Read the model definition and answer for the solid it produces. Units are mm, in the model's axes. A direction names the side the tool comes from. Coordinates: 2 decimals unless noted, no trailing zeros. Write each loop counter-clockwise with the first axis right and the second up, starting at its lowest first coordinate (ties: lowest second). Pieces come first, ordered by that corner, then holes. Notation, with made-up numbers: (-0.75, -18.75) -> (40.25, -18.75) arc R20 ccw to (40.25, -2.75) -> close; hole circle Ø2 at (26.5, -27). An arc over 180 degrees is marked (long way). Answer in a Markdown table with one row per item. Add a question column.
Item 1: Given pin 1 Ø7.5 at (x, z) = (141, 517.5) entering from +Y; pin 2 Ø2 at (x, z) = (90, 215.5) entering from +Y, each flat-ended and moving along its own axis, determine where each tip first touches the part or whether it passes through.
Item 2: Straight lines are drawn through the part: line 1 (Z direction, x = 42, y = 195); line 2 (Y direction, x = 225, z = 163.5); line 3 (Z direction, x = 191, y = 358.5). For each, find the intervals that lie inside material, in ascending order. Write a range as from..to.
Item 3: For a pull along Z with two mould halves and no side action, classify faces 4 (the face through (188, 0, 263)), 5 (the face through (188, 175, 0)), 6 (the face through (188, 168, 533.4)) as +Z half, -Z half, draft (parallel to the pull), parting line (faces both ways), or undercut.
Item 4: Which of the six approach directions +Z, -Z, +X, -X, +Y, -Y give full straight-line access (tool end or side, diameter ignored) to faces 1 (the face through (188, 381, 13)), 2 (the face through (188, 193, 25.4)), 3 (the face through (188, 355.6, 521))?
Item 5: Section B-B on x = 97.5 is taken. Write down the section's boundary in (y, z), then the cut area to 3 significant figures.
Item 6: Section C-C on z = 370 is taken. Write down the section's boundary in (x, y), then the cut area to 3 significant figures.
Item 7: Section A-A on y = 272 is taken. Write down the section's boundary in (x, z), then the cut area to 3 significant figures.
```python
from build123d import *

# Parameters (mm, degrees)
F0_W     = 381
F0_H     = 381
F1_DEPTH = 25.4
F2_W     = 25.4
F2_H     = 508
F3_DEPTH = 381
F4_W     = 381
F4_H     = 355.6
F4_H_2   = 25.4
F5_DEPTH = 25.4


with BuildPart() as f1:
    # F0 (on Top) → F1 (new body)
    with BuildSketch(Plane.XY):
        with Locations((190.5, 190.5)):
            Rectangle(F0_W, F0_H)
    extrude(amount=F1_DEPTH)

    # F2 (on Right) → F3 (join)
    with BuildSketch(Plane.YZ):
        with Locations((-12.7, 254)):
            Rectangle(F2_W, F2_H)
    extrude(amount=F3_DEPTH)

    # F4 (on face) → F5 (join)
    with BuildSketch(Plane.XY.offset(508)):
        with Locations((190.5, 177.8)):
            Rectangle(F4_W, F4_H)
        with Locations((190.5, -12.7)):
            Rectangle(F4_W, F4_H_2)
    extrude(amount=F5_DEPTH)


solid = f1.part
```
Results below:
| question | item | result |
|---|---|---|
| 1 | pin 1 | stops at y = 355.6 |
| 1 | pin 2 | stops at y = 0 |
| 2 | line 1 | z = 0..25.4, 508..533.4 |
| 2 | line 2 | y = -25.4..0 |
| 2 | line 3 | z = 0..25.4 |
| 3 | face 4 | undercut |
| 3 | face 5 | -Z half |
| 3 | face 6 | +Z half |
| 4 | face 1 | +Z, -Z, +X, -X, +Y |
| 4 | face 2 | +X, -X, +Y |
| 4 | face 3 | +Z, +X, -X, +Y |
| 5 | outline | (-25.4, 0) -> (381, 0) -> (381, 25.4) -> (0, 25.4) -> (0, 508) -> (355.6, 508) -> (355.6, 533.4) -> (-25.4, 533.4) -> close |
| 5 | area | 32,300 mm2 |
| 6 | outline | (0, -25.4) -> (381, -25.4) -> (381, 0) -> (0, 0) -> close |
| 6 | area | 9,680 mm2 |
| 7 | outline | (0, 0) -> (381, 0) -> (381, 25.4) -> (0, 25.4) -> close; (0, 508) -> (381, 508) -> (381, 533.4) -> (0, 533.4) -> close |
| 7 | area | 19,400 mm2 |
